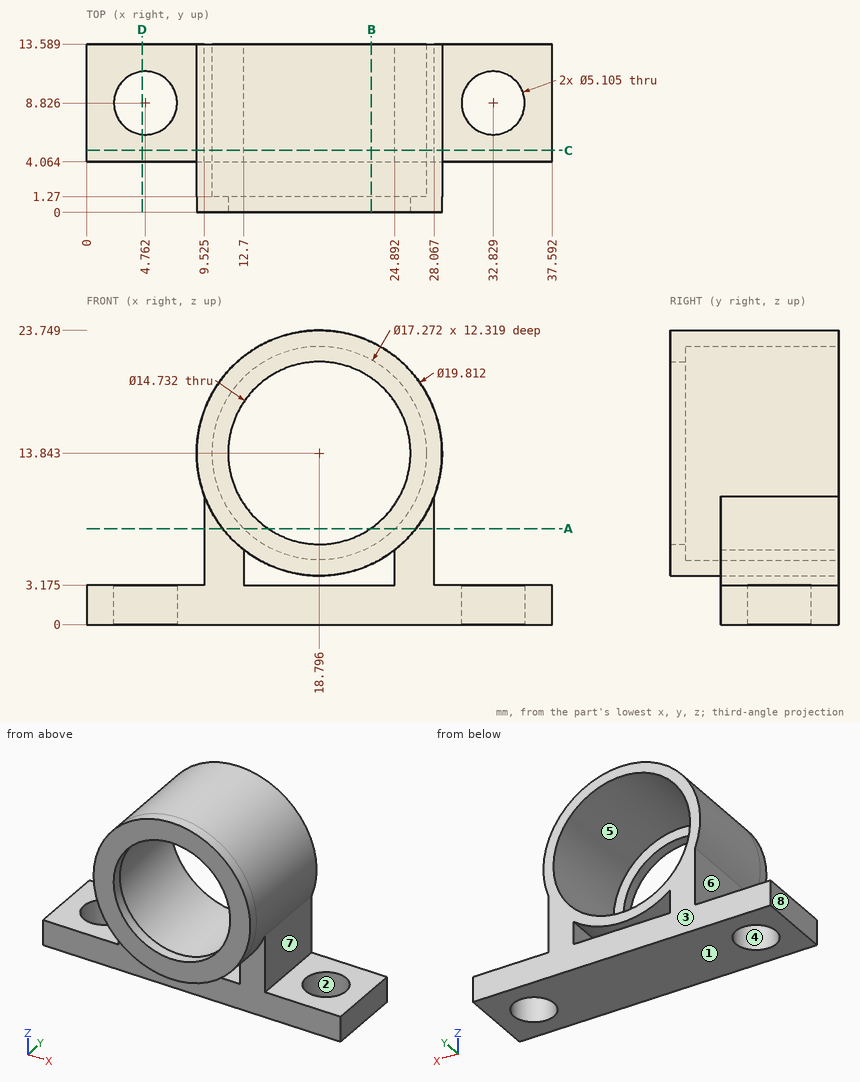
Source: three-view drawing plus pictorial views. Frame: mm from the lowest corner of the part. A direction names the side the tool comes from. Give positions to 0.01 mm unless a question says otherwise; leave off trailing zeros. Order: outer loops, then holes, each group sorted by start corner. A loop starts at its lowest first (then second) coordinate and runs counter-clockwise, first axis right, second up. Notation, with made-up numbers: (1.25, -8.75) -> (24.25, -8.75) arc R27 ccw to (24.25, 27.25) -> close; hole circle Ø2 at (18.25, 81.5). An arc over 180 degrees is marked (long way). Write each question's results on one line, items separated by ' | '. Start each with the question number.
Item 1: Line query: line 1 (Y direction, x = 14, z = 1.5) (1 decimal); line 2 (X direction, y = 6, z = 12.5) (1 decimal); line 3 (X direction, y = 10, z = 8.75) (1 decimal). Output: solid intervals per line, ascending.
Item 2: Set-up query: the marked faces 5, 6, 7 and 8. Return all of +Z, -Z, +X, -X, +Y, -Y with unobstructed straight access to the full face (end or side cutting, diameter ignored); none if empty.
Item 3: Cut plane A-A on z = 7.75. Return the cut outline in (x, y) (1 decimal).
Item 4: Contact query for flat-ended pins moving along their axis: P1, Ø8, axis at y = 7.5, z = 21, coming from the +X side (1 decimal); P2, Ø5, axis at x = 33, y = 7.5, coming from the +Z side (1 decimal); P3, Ø1.5, axis at x = 17, z = 9, coming from the -Y side; P4, Ø3.5, axis at y = 8.5, z = 7, coming from the +X side. Output: stop coordinate, or through.
Item 5: Cut plane B-B on x = 23. Return the cut outline in (y, z) (1 decimal).
Item 6: Cut plane D-D on x = 4.5. Return the cut outline in (y, z) (1 decimal), then the cut area to 3 significant figures.
Item 7: Cut plane C-C on y = 5. Return the cut outline in (x, z) (1 decimal).
Item 8: Mould query, pull axis Y, two halves, no side actions, for the marked faces 1, 2, 3 and 4. Classes: pulls with the +Y half, pulls with the -Y half, needs draft (parallel to the pull), parting line crosses it, or undercut.
Established:
1) line 1: 4.1 to 13.6 | line 2: 9 to 10.3, 27.3 to 28.6 | line 3: 9.5 to 11.8, 25.8 to 28.1
2) face 5: +Y | face 6: -X, +Y, -Y | face 7: +X, +Y, -Y | face 8: +Z, -Z, -X, +Y, -Y
3) outline: (9.5, 4.1) -> (11, 4.1) -> (11, 0) -> (14.7, 0) -> (14.7, 1.3) -> (12.7, 1.3) -> (12.7, 13.6) -> (9.5, 13.6) -> close; (22.9, 0) -> (26.6, 0) -> (26.6, 4.1) -> (28.1, 4.1) -> (28.1, 13.6) -> (24.9, 13.6) -> (24.9, 1.3) -> (22.9, 1.3) -> close
4) P1: x = 28.2 | P2: z = 3.2 | P3: through | P4: x = 28.07
5) outline: (0, 4.9) -> (13.6, 4.9) -> (13.6, 6.3) -> (1.3, 6.3) -> (1.3, 7.8) -> (0, 7.8) -> close; (0, 19.9) -> (1.3, 19.9) -> (1.3, 21.4) -> (13.6, 21.4) -> (13.6, 22.8) -> (0, 22.8) -> close; (4.1, 0) -> (13.6, 0) -> (13.6, 3.2) -> (4.1, 3.2) -> close
6) outline: (4.1, 0) -> (6.3, 0) -> (6.3, 3.2) -> (4.1, 3.2) -> close; (11.4, 0) -> (13.6, 0) -> (13.6, 3.2) -> (11.4, 3.2) -> close | area: 14.1 mm^2
7) outline: (0, 0) -> (37.6, 0) -> (37.6, 3.2) -> (28.1, 3.2) -> (28.1, 10.4) arc R9.9 ccw (long way) to (9.5, 10.4) -> (9.5, 3.2) -> (0, 3.2) -> close; hole circle Ø17.3 at (18.8, 13.8); hole (12.7, 3.2) -> (24.9, 3.2) -> (24.9, 6) arc R9.9 cw to (12.7, 6) -> close
8) face 1: needs draft | face 2: undercut | face 3: pulls with the +Y half | face 4: undercut
